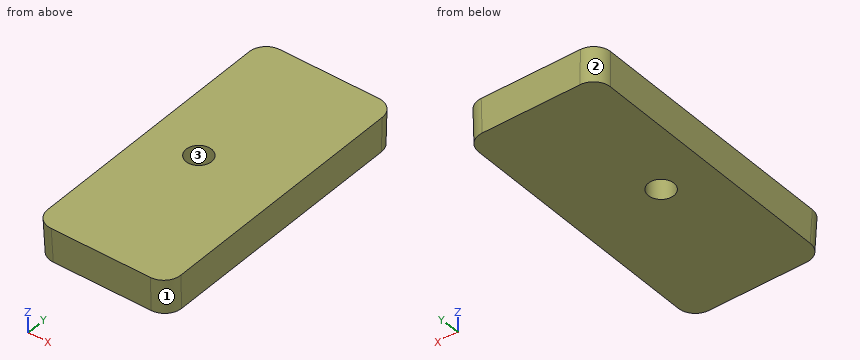
Autodesk Inventor part; units mm, degrees
ref_plane "YZ Plane" through (0, 0, 0) normal (1, 0, 0) x (0, 1, 0)
ref_plane "XZ Plane" through (0, 0, 0) normal (0, 1, 0) x (-1, 0, 0)
ref_plane "XY Plane" through (0, 0, 0) normal (0, 0, 1) x (1, 0, 0)
ref_plane "Arbeitsebene1" through (0, 0, 0) normal (0, 0, 1) x (1, 0, 0)
sketch "Skizze1" plane through (0, 0, 0) normal (0, 0, 1) x (1, 0, 0)
  line L0 (20.3781, -18.1328) -> (23.4454, -18.9546) construction
  line L1 (23.4454, -18.9546) -> (24.2672, -22.0219) construction
  line L2 (24.2672, -22.0219) -> (22.0219, -24.2672) construction
  line L3 (22.0219, -24.2672) -> (18.9546, -23.4454) construction
  line L4 (18.9546, -23.4454) -> (18.1328, -20.3781) construction
  line L5 (18.1328, -20.3781) -> (20.3781, -18.1328) construction
  line L6 (-24.2672, 22.0219) -> (-22.0219, 24.2672) construction
  line L7 (-22.0219, 24.2672) -> (-18.9546, 23.4454) construction
  line L8 (-18.9546, 23.4454) -> (-18.1328, 20.3781) construction
  line L9 (-18.1328, 20.3781) -> (-20.3781, 18.1328) construction
  line L10 (-20.3781, 18.1328) -> (-23.4454, 18.9546) construction
  line L11 (-23.4454, 18.9546) -> (-24.2672, 22.0219) construction
  circle A0 centre (20.66, 14.3) radius 2.475 construction
  circle A1 centre (14.3, -20.66) radius 2.475 construction
  circle A2 centre (-20.66, -14.3) radius 2.475 construction
  circle A3 centre (-14.3, 20.66) radius 2.475 construction
  circle A4 centre (14.3, 20.66) radius 2.475 construction
  circle A5 centre (-20.66, 14.3) radius 2.475 construction
  circle A6 centre (-14.3, -20.66) radius 2.475 construction
  circle A7 centre (20.66, -14.3) radius 2.475 construction
  arc A8 (-8.8, -18.96) -> (-8.8, -22.36) centre (-8.8, -20.66) ccw construction
  line L12 (-8.8, -18.96) -> (8.8, -18.96) construction
  arc A9 (8.8, -22.36) -> (8.8, -18.96) centre (8.8, -20.66) ccw construction
  line L13 (8.8, -22.36) -> (-8.8, -22.36) construction
  arc A10 (-8.8, 22.36) -> (-8.8, 18.96) centre (-8.8, 20.66) ccw construction
  line L14 (-8.8, 22.36) -> (8.8, 22.36) construction
  arc A11 (8.8, 18.96) -> (8.8, 22.36) centre (8.8, 20.66) ccw construction
  line L15 (8.8, 18.96) -> (-8.8, 18.96) construction
  arc A12 (-18.96, 8.8) -> (-22.36, 8.8) centre (-20.66, 8.8) ccw construction
  line L16 (-18.96, 8.8) -> (-18.96, -8.8) construction
  arc A13 (-22.36, -8.8) -> (-18.96, -8.8) centre (-20.66, -8.8) ccw construction
  line L17 (-22.36, -8.8) -> (-22.36, 8.8) construction
  arc A14 (18.96, -8.8) -> (22.36, -8.8) centre (20.66, -8.8) ccw construction
  line L18 (18.96, -8.8) -> (18.96, 8.8) construction
  arc A15 (22.36, 8.8) -> (18.96, 8.8) centre (20.66, 8.8) ccw construction
  line L19 (22.36, 8.8) -> (22.36, -8.8) construction
  line L20 (-16.97, -16.97) -> (-16.97, 16.97) construction
  line L21 (-16.97, 16.97) -> (16.97, 16.97) construction
  line L22 (16.97, 16.97) -> (16.97, -16.97) construction
  line L23 (16.97, -16.97) -> (-16.97, -16.97) construction
  circle A16 centre (-21.2, -21.2) radius 2.75 construction
  circle A17 centre (21.2, 21.2) radius 2.75 construction
  arc A18 (-24.35, -22.85) -> (-22.85, -24.35) centre (-22.85, -22.85) ccw construction
  line L24 (22.85, -24.35) -> (-22.85, -24.35) construction
  arc A19 (22.85, -24.35) -> (24.35, -22.85) centre (22.85, -22.85) ccw construction
  line L25 (24.35, 22.85) -> (24.35, -22.85) construction
  arc A20 (24.35, 22.85) -> (22.85, 24.35) centre (22.85, 22.85) ccw construction
  line L26 (-22.85, 24.35) -> (22.85, 24.35) construction
  arc A21 (-22.85, 24.35) -> (-24.35, 22.85) centre (-22.85, 22.85) ccw construction
  line L27 (-24.35, -22.85) -> (-24.35, 22.85) construction
  line L28 (-16.97, 16.97) -> (16.97, 16.97)
  line L29 (16.97, 16.97) -> (16.97, -16.97)
  line L30 (16.97, -16.97) -> (-16.97, -16.97)
  line L31 (-16.97, -16.97) -> (-16.97, 16.97)
  point P0 (0, 0)
extrude "Extrusion1" add sketch "Skizze1" against normal blind 4 draft -2
sketch "Skizze2" plane through (0, 0, 0) normal (0, 0, 1) x (1, 0, 0)
  circle A0 centre (-11.03, 0) radius 2.5
  circle A1 centre (-11.03, 0) radius 1.5
  point P0 (0, 0)
  dimension "d3" = 3
extrude "Extrusion2" cut sketch "Skizze2" against normal blind 4 contours A1
fillet "Rundung1" radius 2 4 edges at (-16.9002, -16.9002, -2) (16.9002, -16.9002, -2) (16.9002, 16.9002, -2) (-16.9002, 16.9002, -2)
sketch "Skizze3" plane through (0, 0, 0) normal (0, 0, 1) x (1, 0, 0)
  circle A0 centre (28.0867, -9.6825) radius 1.4 construction
  circle A1 centre (33.0867, 9.6314) radius 1.4 construction
  circle A2 centre (33.0867, -9.6825) radius 1.4 construction
  circle A3 centre (28.0867, 9.6314) radius 1.4 construction
  circle A4 centre (-11.03, 0) radius 3 construction
  circle A5 centre (0.47, 11.5) radius 1.75 construction
  circle A6 centre (0.47, -11.5) radius 1.75 construction
  line L0 (14.4713, 6.5256) -> (36.5731, 6.5256) construction
  line L1 (36.5731, 16.4952) -> (36.5731, 6.5256) construction
  line L2 (-2.8633, 16.4952) -> (36.5731, 16.4952) construction
  line L3 (-24.53, 3.4952) -> (-2.8633, 16.4952) construction
  line L4 (-24.53, 3.4952) -> (-24.53, -3.4952) construction
  line L5 (-24.53, -3.4952) -> (-2.8633, -16.4952) construction
  line L6 (-2.8633, -16.4952) -> (36.5731, -16.4952) construction
  line L7 (36.5731, -16.4952) -> (36.5731, -6.4744) construction
  line L8 (36.5731, -6.4744) -> (14.4713, -6.4744) construction
  line L9 (14.4713, -6.4744) -> (14.4713, -13.5) construction
  line L10 (14.4713, -13.5) -> (4.1713, -13.5) construction
  line L11 (4.1713, -13.5) -> (4.1713, 13.5) construction
  line L12 (4.1713, 13.5) -> (14.4713, 13.5) construction
  line L13 (14.4713, 13.5) -> (14.4713, 6.5256) construction
  circle A7 centre (-11.03, 0) radius 1.5 construction
  ellipse E0 centre (-14.9688, 14.9688) end of major axis (-16.3847, 16.3847) minor radius 2 (-14.9712, 16.97) -> (-16.97, 14.9712) ccw construction
  line L14 (-16.97, 14.9712) -> (-16.97, -14.9712) construction
  ellipse E1 centre (-14.9688, -14.9688) end of major axis (-16.3847, -16.3847) minor radius 2 (-16.97, -14.9712) -> (-14.9712, -16.97) ccw construction
  line L15 (-14.9712, -16.97) -> (14.9712, -16.97) construction
  ellipse E2 centre (14.9688, -14.9688) end of major axis (16.3847, -16.3847) minor radius 2 (14.9712, -16.97) -> (16.97, -14.9712) ccw construction
  line L16 (16.97, -14.9712) -> (16.97, 14.9712) construction
  ellipse E3 centre (14.9688, 14.9688) end of major axis (16.3847, 16.3847) minor radius 2 (16.97, 14.9712) -> (14.9712, 16.97) ccw construction
  line L17 (14.9712, 16.97) -> (-14.9712, 16.97) construction
  line L18 (-14.8315, -16.8303) -> (14.8315, -16.8303)
  line L19 (16.97, 16.97) -> (-1.28, 16.97)
  line L20 (-1.28, 16.97) -> (-1.28, -16.8303)
  line L21 (-1.28, -16.8303) -> (16.97, -16.8303)
  line L22 (16.97, -16.8303) -> (16.97, 16.97)
  line L23 (-14.9712, -16.97) -> (14.9712, -16.97)
  line L24 (16.97, -16.8303) -> (-1.28, -16.8303)
  line L25 (-1.28, -16.8303) -> (-1.28, -16.97)
  line L26 (-1.28, -16.97) -> (16.97, -16.97)
  line L27 (16.97, -16.97) -> (16.97, -16.8303)
  point P0 (0, 0)
  point P1 (14.8315, -16.8303)
extrude "Extrusion3" cut sketch "Skizze3" against normal blind 4
fillet "Rundung2" radius 2 2 edges at (-1.28, -16.9002, -2) (-1.28, 16.9002, -2)
properties part number "30_Cube_Z_Focus_MGN_NEMA_counterplate_inner"
For this review, take the finished solid that the model builds, in its own axes (mm). Face numbers are marked on the shaded views. Round coordinates to 2 decimals unless told otherwise and drop trailing zeros. Write each loop counter-clockwise with the first axis right and the second up, starting at its lowest first coordinate (ties: lowest second). Pieces come first, ordered by that corner, then holes. Notation, with made-up numbers: (-5.75, -14.5) - (21.25, -14.5) arc R25 cw to (21.25, 23.5) - close; hole circle Ø1 at (40, 80). An arc over 180 degrees is marked (long way). Use a Markdown table: item, result.
Q1. Wall thickness on line 1 along X through (y, z) = (-1, -0.6); line 2 along Y through (x, z) = (-11.03, -2.3); line 3 along Y through (x, z) = (-9.75, -2): over which ranges is each line inside the solid? List them lowest first.
Derived:
| item | result |
|---|---|
| line 1 | x = -16.95 to -12.15, -9.91 to -1.28 |
| line 2 | y = -16.89 to -1.5, 1.5 to 16.89 |
| line 3 | y = -16.9 to -0.78, 0.78 to 16.9 |
Q2. The part is to be moulded in two halves that separate along X. For the marked faces 1, 2 and 3, say which applies: pulls with the +X half, pulls with the -X half, needs draft (parallel to the pull), parting line crosses it, or undercut.
Derived:
| item | result |
|---|---|
| face 1 | pulls with the +X half |
| face 2 | pulls with the -X half |
| face 3 | undercut |
Q3. We need section A-A (y = 0). Give the boundary of the cut face in (x, z).
Derived:
| item | result |
|---|---|
| outline | (-16.97, 0) - (-16.83, -4) - (-12.53, -4) - (-12.53, 0) - close; (-9.53, -4) - (-1.28, -4) - (-1.28, 0) - (-9.53, 0) - close |
Q4. We need section B-B (x = -11.03). Give the boundary of the cut face in (y, z), plus the area to 3 significant figures.
Derived:
| item | result |
|---|---|
| outline | (-16.97, 0) - (-16.83, -4) - (-1.5, -4) - (-1.5, 0) - close; (1.5, -4) - (16.83, -4) - (16.97, 0) - (1.5, 0) - close |
| area | 123 mm2 |
Q5. Clearance check with flat-ended pins moving along their axes: pin 1 (1 mm diameter, centred on x = -11.5, z = -1, fed in from -Y); pin 2 (2.5 mm diameter, centred on x = -11.03, y = 0, fed in from +Z). State where each tip first meets the part, or that it passes through.
Derived:
| item | result |
|---|---|
| pin 1 | stops at y = -16.95 |
| pin 2 | passes through |
